Work out the finished part from the listing and answer in its coordinate system (mm). Face numbers are marked on the shaded views. A direction names the side the tool comes from. Give positions to 0.01 mm unless a question says otherwise; leave off trailing zeros. Loops run counter-clockwise (first coordinate to the right, second up) from the corner with the lowest first, then second, coordinate; pieces in that order, holes last. Notation, with made-up numbers: (67.5, 20.25) - (84.5, 20.25) arc R26 cw to (84.5, 35.25) - close; hole circle Ø3 at (74.25, -9). An arc over 180 degrees is marked (long way). One line per question, with ' | ' between items.
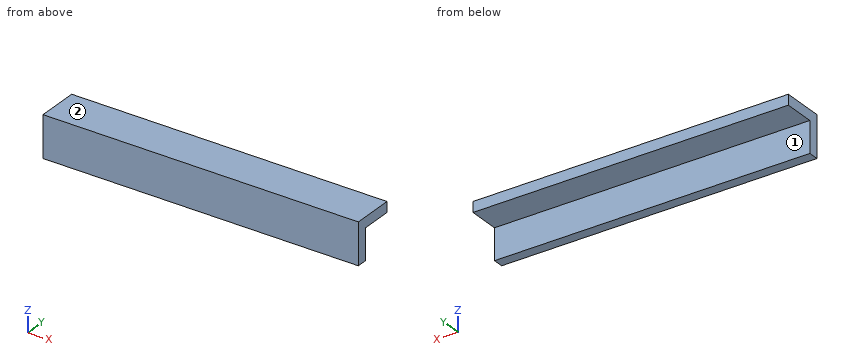
from build123d import *

# Parameters (mm, degrees)
SKETCH1_W           = 96.52
SKETCH1_H           = 12.7
BOSS_EXTRUDE1_DEPTH = 3.175
SKETCH7_W           = 96.52
SKETCH7_H           = 9.525
BOSS_EXTRUDE2_DEPTH = 3.175


with BuildPart() as part:
    # Sketch1 → Boss-Extrude1 (new body)
    with BuildSketch(Plane.XY):
        with Locations((23.526472643, 22.354273404)):
            Rectangle(SKETCH1_W, SKETCH1_H)
    extrude(amount=BOSS_EXTRUDE1_DEPTH)

    # Sketch7 → Boss-Extrude2 (add)
    with BuildSketch(Plane(origin=(0, 16.004273404, 0), x_dir=(-1, 0, 0), z_dir=(0, -1, 0))):
        with Locations((-23.526472643, 4.7625)):
            Rectangle(SKETCH7_W, SKETCH7_H)
    extrude(amount=-BOSS_EXTRUDE2_DEPTH)


solid = part.part
1. Find section B-B on z = -2.75. Write down the section's boundary in (x, y), then the cut area to 3 significant figures.
Evaluation:
outline: (-24.73, 16) - (71.79, 16) - (71.79, 19.18) - (-24.73, 19.18) - close | area: 306 mm2
2. Find section A-A on x = -1.5. Write down the section's boundary in (y, z) (3 decimals), then the cut area to 3 significant figures.
Evaluation:
outline: (16.004, -9.525) - (19.179, -9.525) - (19.179, 0) - (28.704, 0) - (28.704, 3.175) - (16.004, 3.175) - close | area: 70.6 mm2
3. Consider L1, parallel to Z at x = 8.5, y = 26 (3 decimals); L2, parallel to Y at x = 52.5, z = -5.5. Determine where each line is inside the solid, lowest interval first.
Evaluation:
L1: 0 to 3.175 | L2: 16 to 19.18
4. Find section C-C on y = 26.5. Write down the section's boundary in (x, z) (3 decimals).
Evaluation:
outline: (-24.734, 0) - (71.786, 0) - (71.786, 3.175) - (-24.734, 3.175) - close
5. Which of the six approach directions +Z, -Z, +X, -X, +Y, -Y give full straight-line access (tool end or side, diameter ignored) to the marked faces 1 and 2?
Evaluation:
face 1: -Z, +X, -X, +Y | face 2: +Z, +X, -X, +Y, -Y
6. Flat-ended cylindrical pins translate along their axes: pin 1 (5 mm diameter, centred on x = 35, z = -7, fed in from +Y); pin 2 (5 mm diameter, centred on x = 29.5, y = 24.5, fed in from -Z). Find the tip coordinate at first contact, or state that the pin passes through.
Evaluation:
pin 1: y = 19.18 | pin 2: z = 0
